```python
from build123d import *

# Parameters (mm, degrees)
F0_W     = 600
F0_H     = 150
F0_W_2   = 590
F0_H_2   = 140
F1_DEPTH = 5
F2_W     = 600
F2_H     = 150
F3_DEPTH = 1
F4_DEPTH = 1


with BuildPart() as f1:
    # F0 (on Top) → F1 (new body)
    with BuildSketch(Plane.XY):
        with Locations((11.197913, -43.259316)):
            Rectangle(F0_W, F0_H)
        with Locations((11.197913, -43.259316)):
            Rectangle(F0_W_2, F0_H_2, mode=Mode.SUBTRACT)
    extrude(amount=F1_DEPTH)

    # F2 (on face) → F3 (join)
    with BuildSketch(Plane(origin=(0, 0, 0), x_dir=(1, 0, 0), z_dir=(0, 0, -1))):
        with Locations((11.197913, 43.259316)):
            Rectangle(F2_W, F2_H)
    extrude(amount=F3_DEPTH)

    # F0 (on Top) → F4 (join)
    with BuildSketch(Plane.XY):
        with Locations((11.197913, -43.259316)):
            Rectangle(F0_W, F0_H)
        with Locations((11.197913, -43.259316)):
            Rectangle(F0_W_2, F0_H_2, mode=Mode.SUBTRACT)
    extrude(amount=F4_DEPTH)


solid = f1.part
```
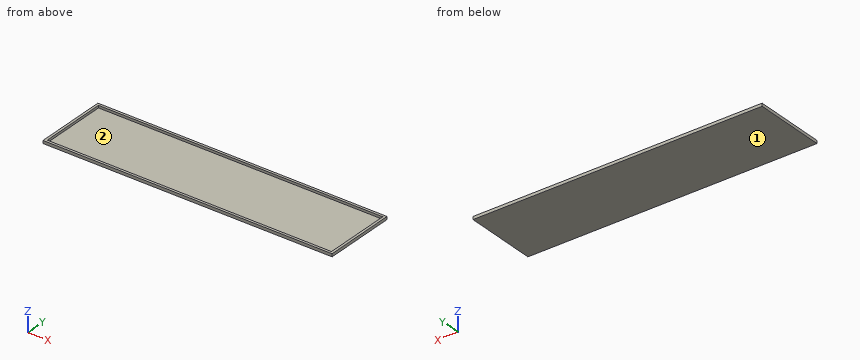
Geometry check sheet. Reference: the model listing, model coordinates, mm. Face numbers are marked on the shaded views. Coordinates: 2 decimals unless noted, no trailing zeros. Loops run counter-clockwise (first coordinate to the right, second up) from the corner with the lowest first, then second, coordinate; pieces in that order, holes last. Notation, with made-up numbers: (40.5, -32.75) -> (66.5, -32.75) arc R24 ccw to (66.5, -17.75) -> close; hole circle Ø7 at (60.25, 23.25). An arc over 180 degrees is marked (long way). Put each result on its own line as item: value.
1) Release check for a two-part mould opening along Y. For the marked faces 1 and 2 record: released by +Y, released by -Y, zero draft, split by the parting line, or undercut.
Result set:
face 1: zero draft
face 2: undercut
2) Cross-section at C-C on x = -121. Record the boundary of the cut face in (y, z), plus the area to 3 significant figures.
Result set:
outline: (-118.26, -1) -> (31.74, -1) -> (31.74, 5) -> (26.74, 5) -> (26.74, 0) -> (-113.26, 0) -> (-113.26, 5) -> (-118.26, 5) -> close
area: 200 mm^2
3) Gauge pin test, flat end, axial feed: pin 1 Ø2 at (x, y) = (-177.5, -22.5) entering from +Z. Record the tip position at first contact, or that the pin passes through.
Result set:
pin 1: stops at z = 0
4) Cross-section at A-A on y = -41.5. Record the boundary of the cut face in (x, z), plus the area to 3 significant figures.
Result set:
outline: (-288.8, -1) -> (311.2, -1) -> (311.2, 5) -> (306.2, 5) -> (306.2, 0) -> (-283.8, 0) -> (-283.8, 5) -> (-288.8, 5) -> close
area: 650 mm^2
5) Thickness scan on line 1 (Y direction, x = 287.5, z = 4.75); line 2 (X direction, y = 23.5, z = 0.65); line 3 (Z direction, x = -18, y = -4). Record the ranges inside material, lowest first.
Result set:
line 1: y = -118.26 to -113.26, 26.74 to 31.74
line 2: x = -288.8 to -283.8, 306.2 to 311.2
line 3: z = -1 to 0
6) Cross-section at B-B on z = 3.05. Record the boundary of the cut face in (x, y).
Result set:
outline: (-288.8, -118.26) -> (311.2, -118.26) -> (311.2, 31.74) -> (-288.8, 31.74) -> close; hole (-283.8, -113.26) -> (306.2, -113.26) -> (306.2, 26.74) -> (-283.8, 26.74) -> close
